Build history of the part. All positions in model axes, mm. Face numbers are marked on the shaded views. A direction names the side the tool comes from. Coordinates: 2 decimals unless noted, no trailing zeros. Loops run counter-clockwise (first coordinate to the right, second up) from the corner with the lowest first, then second, coordinate; pieces in that order, holes last.
Item 1: Cut at D-D (x = 60.5). List the corners of the cut face in (y, z).
Item 2: 3-axis set-ups, long thin cutter, end or side, ignore diameter. For the marked faces 5 and 6: which of +Z, -Z, +X, -X, +Y, -Y reach the whole face in a straight line?
Item 3: Mould opens along X. For the marked faces 1, 2, 3 and 4 say: released by +X, released by -X, zero draft, split by the parting line, or undercut.
Item 4: Drill centre lines: line 1 along X through (y, z) = (25, 1.5); line 2 along Y through (x, z) = (24, 2.05); line 3 along X through (y, z) = (51, 0.5). Where is each one in solid material? Low to high.
Item 5: Flat gauge pins, fed straight in: pin 1 (2.5 mm diameter, centred on x = 7, z = 1.5, fed in from -Y); pin 2 (2.5 mm diameter, centred on y = 12.5, z = 1.5, fed in from +X); pin 3 (1.5 mm diameter, centred on x = 45, z = 2, fed in from -Y); pin 4 (2.5 mm diameter, centred on y = 68, z = 2, fed in from -X). Where does each tip first touch, or does it go through?
Item 6: Cut at B-B (z = 2.3). List the corners of the cut face in (x, y).
Item 7: Cut at A-A (y = 12.5). List the corners of the cut face in (x, z).
Item 8: Cut at C-C (y = 46). List the corners of the cut face in (x, z).
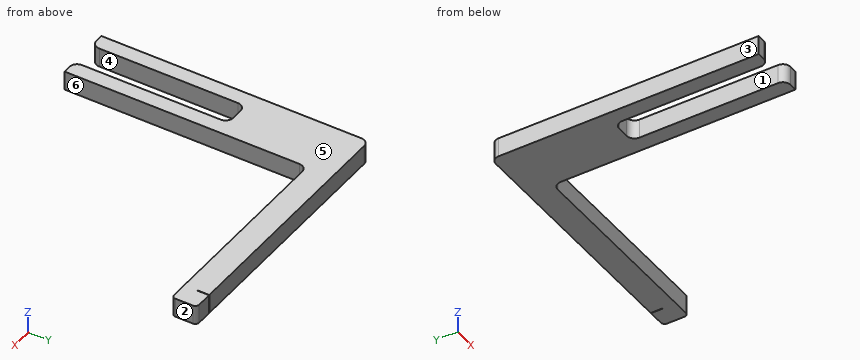
from build123d import *

# Parameters (mm, degrees)
BOSS_EXTRUDE1_DEPTH = 5
SKETCH3_W           = 0.1
SKETCH3_H           = 5
CUT_EXTRUDE1_DEPTH  = 3
FILLET1_R           = 2


with BuildPart() as part:
    # Sketch1 → Boss-Extrude1 (new body)
    with BuildSketch(Plane.XY):
        with BuildLine():
            Line((0, 0), (0, 67.5))
            ThreePointArc((0, 67.5), (0.585786438, 68.914213562), (2, 69.5))
            Line((2, 69.5), (69, 69.5))
            ThreePointArc((69, 69.5), (69.707106781, 69.207106781), (70, 68.5))
            Line((70, 68.5), (70, 64))
            ThreePointArc((70, 64), (69.707106781, 63.292893219), (69, 63))
            Line((69, 63), (17, 63))
            ThreePointArc((17, 63), (15.585786438, 62.414213562), (15, 61))
            Line((15, 61), (15, 0))
            Line((15, 0), (11, 0))
            Line((11, 0), (11, 40))
            Line((11, 40), (4, 40))
            Line((4, 40), (4, 0))
            Line((4, 0), (0, 0))
        make_face()
    extrude(amount=BOSS_EXTRUDE1_DEPTH)

    # Sketch3 → Cut-Extrude1 (cut)
    with BuildSketch(Plane(origin=(0, 69.5, 0), x_dir=(1, 0, 0), z_dir=(0, 1, 0))):
        with Locations((64.95, -2.5)):
            Rectangle(SKETCH3_W, SKETCH3_H)
    extrude(amount=-CUT_EXTRUDE1_DEPTH, mode=Mode.SUBTRACT)

    # Fillet1
    fillet1_edges = [part.edges().sort_by_distance(p)[0] for p in [
        (11, 0, 2.5),
        (11, 40, 2.5),
        (4, 40, 2.5),
        (4, 0, 2.5),
    ]]
    fillet(fillet1_edges, radius=FILLET1_R)


solid = part.part
Filled sheet:
1. outline: (63, 0) - (69.5, 0) - (69.5, 5) - (63, 5) - close
2. face 5: +Z, +X, -X, +Y, -Y
2. face 6: +Z, -Z, +X, -Y
3. face 1: undercut
3. face 2: released by +X
3. face 3: released by -X
3. face 4: undercut
4. line 1: x = 0 to 4, 11 to 15
4. line 2: y = 63 to 69.5
4. line 3: x = 0 to 15
5. pin 1: stops at y = 39.98
5. pin 2: stops at x = 15
5. pin 3: stops at y = 63
5. pin 4: stops at x = 0
6. outline: (0, 0) - (2, 0) arc R2 ccw to (4, 2) - (4, 38) arc R2 cw to (6, 40) - (9, 40) arc R2 cw to (11, 38) - (11, 2) arc R2 ccw to (13, 0) - (15, 0) - (15, 61) arc R2 cw to (17, 63) - (69, 63) arc R1 ccw to (70, 64) - (70, 68.5) arc R1 ccw to (69, 69.5) - (65, 69.5) - (65, 66.5) - (64.9, 66.5) - (64.9, 69.5) - (2, 69.5) arc R2 ccw to (0, 67.5) - close
7. outline: (0, 0) - (4, 0) - (4, 5) - (0, 5) - close; (11, 0) - (15, 0) - (15, 5) - (11, 5) - close
8. outline: (0, 0) - (15, 0) - (15, 5) - (0, 5) - close
